For this review, take the finished solid that the model builds, in its own axes (mm). A direction names the side the tool comes from. Round coordinates to 2 decimals unless told otherwise and drop trailing zeros. Order: outer loops, then holes, each group sorted by start corner. A loop starts at its lowest first (then second) coordinate and runs counter-clockwise, first axis right, second up. Notation, with made-up numbers: M 45.25,86.25 L 61.25,86.25 A31 ccw 61.25,113.25 Z; hole C -10.75,-14.75 d4. An arc over 180 degrees is marked long. Use a Markdown table: item, result.
from build123d import *

# Parameters (mm, degrees)
F1_DEPTH = 10


with BuildPart() as f1:
    # F0 (on Front) → F1 (new body)
    with BuildSketch(Plane.XZ):
        with BuildLine():
            ThreePointArc((0, 5), (3.535534, 3.535534), (5, 0))
            Line((5, 0), (25, 0))
            Line((25, 0), (25, 10))
            Line((25, 10), (40, 10))
            Line((40, 10), (40, 20))
            Line((40, 20), (10, 20))
            Line((10, 20), (10, 15))
            Line((10, 15), (0, 15))
            Line((0, 15), (0, 5))
        make_face()
        with BuildLine():
            Line((25, 0), (5, 0))
            ThreePointArc((5, 0), (3.535534, -3.535534), (0, -5))
            Line((0, -5), (0, -15))
            Line((0, -15), (10, -15))
            Line((10, -15), (10, -20))
            Line((10, -20), (40, -20))
            Line((40, -20), (40, -10))
            Line((40, -10), (25, -10))
            Line((25, -10), (25, 0))
        make_face()
        with BuildLine():
            ThreePointArc((-5, 0), (-3.535534, 3.535534), (0, 5))
            Line((0, 5), (0, 15))
            Line((0, 15), (-10, 15))
            Line((-10, 15), (-10, 20))
            Line((-10, 20), (-40, 20))
            Line((-40, 20), (-40, 10))
            Line((-40, 10), (-25, 10))
            Line((-25, 10), (-25, 0))
            Line((-25, 0), (-25, -10))
            Line((-25, -10), (-40, -10))
            Line((-40, -10), (-40, -20))
            Line((-40, -20), (-10, -20))
            Line((-10, -20), (-10, -15))
            Line((-10, -15), (0, -15))
            Line((0, -15), (0, -5))
            ThreePointArc((0, -5), (-3.535534, -3.535534), (-5, 0))
        make_face()
    extrude(amount=F1_DEPTH)


solid = f1.part
Q1. Wall thickness on line 1 along X through (y, z) = (-3.5, 17); line 2 along Z through (x, y) = (-34, -9); line 3 along X through (y, z) = (-7, 7.5): over which ranges is each line inside the solid? List them lowest first. Write a range as [from, to].
Determined:
| item | result |
|---|---|
| line 1 | x = [-40, -10], [10, 40] |
| line 2 | z = [-20, -10], [10, 20] |
| line 3 | x = [-25, 25] |
Q2. Draft analysis for pull direction Z (two halves, no side actions). For faces 1 (the flat face through (25, -5, 20)), 2 (the flat face through (-10, -5, -18)), 3 (the flat face through (25, -5, 0)), state which applies: pulls with the +Z half, pulls with the -Z half, needs draft (parallel to the pull), parting line crosses it, or undercut.
Determined:
| item | result |
|---|---|
| face 1 | pulls with the +Z half |
| face 2 | needs draft |
| face 3 | undercut |
Q3. Add section A-A (y = -9). Write out the cut boundary in (x, z).
Determined:
| item | result |
|---|---|
| outline | M -40,-20 L -10,-20 L -10,-15 L 10,-15 L 10,-20 L 40,-20 L 40,-10 L 25,-10 L 25,10 L 40,10 L 40,20 L 10,20 L 10,15 L -10,15 L -10,20 L -40,20 L -40,10 L -25,10 L -25,-10 L -40,-10 Z; hole C 0,0 d10 |
Q4. Clearance check with flat-ended pins moving along their axes: pin 1 (3 mm diameter, centred on y = -5, z = -1, fed in from +X); pin 2 (2 mm diameter, centred on x = 0.5, y = -1.5, fed in from +Z); pin 3 (1 mm diameter, centred on x = -5, y = -4.5, fed in from -Z). State where each tip first meets the part, or that it passes through.
Determined:
| item | result |
|---|---|
| pin 1 | stops at x = 25 |
| pin 2 | stops at z = 15 |
| pin 3 | stops at z = -15 |
Q5. Add section D-D (x = 1.5). Write out the cut boundary in (y, z), then the cut area to 3 significant figures.
Determined:
| item | result |
|---|---|
| outline | M -10,-15 L 0,-15 L 0,-4.77 L -10,-4.77 Z; M -10,4.77 L 0,4.77 L 0,15 L -10,15 Z |
| area | 205 mm^2 |
Q6. Add section B-B (x = 31.5). Write out the cut boundary in (y, z), then the cut area to 3 significant figures.
Determined:
| item | result |
|---|---|
| outline | M -10,-20 L 0,-20 L 0,-10 L -10,-10 Z; M -10,10 L 0,10 L 0,20 L -10,20 Z |
| area | 200 mm^2 |
Q7. Add section C-C (z = 6). Write out the cut boundary in (x, y).
Determined:
| item | result |
|---|---|
| outline | M -25,-10 L 25,-10 L 25,0 L -25,0 Z |
Q8. Machinability: for faces 4 (the flat face through (-25, -5, 0)), 5 (the flat face through (10, -5, -17)), 6 (the flat face through (33, -5, -10)), 7 (the flat face through (40, -5, -15)), 8 (the flat face through (10, -5, 18)), which of the approach directions +Z, -Z, +X, -X, +Y, -Y give a long, thin tool a straight path to every point of the face, cutting with its end or side? Answer none if there is none.
Determined:
| item | result |
|---|---|
| face 4 | -X, +Y, -Y |
| face 5 | -Z, +Y, -Y |
| face 6 | +X, +Y, -Y |
| face 7 | +Z, -Z, +X, +Y, -Y |
| face 8 | +Z, +Y, -Y |
